```python
from build123d import *

# Parameters (mm, degrees)
SKETCH1_R           = 12.7
BOSS_EXTRUDE1_DEPTH = 1120
SKETCH3_R           = 12.7
SKETCH3_R_2         = 9.525
CUT_EXTRUDE1_DEPTH  = 25.4
SKETCH4_R           = 12.7
SKETCH4_R_2         = 9.525
CUT_EXTRUDE2_DEPTH  = 25.4
SKETCH5_R           = 19.05
SKETCH5_R_2         = 12.7
BOSS_EXTRUDE2_DEPTH = 129


with BuildPart() as part:
    # Sketch1 → Boss-Extrude1 (new body)
    with BuildSketch(Plane(origin=(0, 0, 0), x_dir=(1, 0, 0), z_dir=(0, 1, 0))):
        Circle(SKETCH1_R)
    extrude(amount=BOSS_EXTRUDE1_DEPTH)

    # Sketch3 → Cut-Extrude1 (cut)
    with BuildSketch(Plane.XZ):
        Circle(SKETCH3_R)
        Circle(SKETCH3_R_2, mode=Mode.SUBTRACT)
    extrude(amount=-CUT_EXTRUDE1_DEPTH, mode=Mode.SUBTRACT)

    # Sketch4 → Cut-Extrude2 (cut)
    with BuildSketch(Plane(origin=(0, 1120, 0), x_dir=(1, 0, 0), z_dir=(0, 1, 0))):
        Circle(SKETCH4_R)
        Circle(SKETCH4_R_2, mode=Mode.SUBTRACT)
    extrude(amount=-CUT_EXTRUDE2_DEPTH, mode=Mode.SUBTRACT)

    # Sketch5 → Boss-Extrude2 (add)
    with BuildSketch(Plane(origin=(0, 753, 0), x_dir=(1, 0, 0), z_dir=(0, 1, 0))):
        Circle(SKETCH5_R)
        Circle(SKETCH5_R_2, mode=Mode.SUBTRACT)
    extrude(amount=-BOSS_EXTRUDE2_DEPTH)


solid = part.part
```
Design review of the part built by this model. Coordinates are the model's own, in mm. A direction names the side the tool comes from. Give positions to 0.01 mm unless a question says otherwise; leave off trailing zeros. Loops run counter-clockwise (first coordinate to the right, second up) from the corner with the lowest first, then second, coordinate; pieces in that order, holes last. Notation, with made-up numbers: M -21,80 L 5,80 A28 ccw 5,115 Z; hole C 21,82.25 d3. An arc over 180 degrees is marked long. Return JSON: item names as keys, results as strings. Group by question number.
Item 1: Tool access review of faces 1 (the cylindrical face through (-7.559, 1107.478, 5.796)), 2 (the flat face through (0, 0, 0)), 3 (the flat face through (5, 25.4, 9)): name each direction out of +Z, -Z, +X, -X, +Y, -Y from which nothing blocks a thin tool from reaching the whole face with its end or side.
Item 2: Insertion check: pin 1 Ø12 at (y, z) = (478.5, 7.5) entering from -X; pin 2 Ø1 at (y, z) = (722, -15) entering from +X; pin 3 Ø3 at (x, z) = (13.5, -1.5) entering from +Y. Each pin has a flat end and moves straight along its axis. Give the tip position at first contact, or say it passes through.
Item 3: We need section C-C (y = 1023.5). Give the boundary of the cut face in (x, z).
Item 4: We need section B-B (x = 3). Give the boundary of the cut face in (y, z).
Item 5: For probe 1 along Y at (x, z) = (2, 12.5); probe 2 along Y at (x, z) = (5, -14); probe 3 along X at (y, z) = (613, -1), list the stretches that pass through material, from the lowest coordinate up.
Item 6: We need section A-A (z = 0). Give the boundary of the cut face in (x, y) (3 decimals), and give its area (3 significant figures).
Output:
{
 "1": {"face 1": "+Y", "face 2": "+Z, -Z, +X, -X, -Y", "face 3": "-Y"},
 "2": {"pin 1": "stops at x = -12.61", "pin 2": "stops at x = 12.36", "pin 3": "stops at y = 1094.6"},
 "3": {"outline": "C 0,0 d25.4"},
 "4": {"outline": "M 0,-9.04 L 25.4,-9.04 L 25.4,-12.34 L 624,-12.34 L 624,-18.81 L 753,-18.81 L 753,-12.34 L 1094.6,-12.34 L 1094.6,-9.04 L 1120,-9.04 L 1120,9.04 L 1094.6,9.04 L 1094.6,12.34 L 753,12.34 L 753,18.81 L 624,18.81 L 624,12.34 L 25.4,12.34 L 25.4,9.04 L 0,9.04 Z"},
 "5": {"probe 1": "y = 25.4 to 1094.6", "probe 2": "y = 624 to 753", "probe 3": "x = -12.66 to 12.66"},
 "6": {"outline": "M -19.05,624 L -12.7,624 L -12.7,25.4 L -9.525,25.4 L -9.525,0 L 9.525,0 L 9.525,25.4 L 12.7,25.4 L 12.7,624 L 19.05,624 L 19.05,753 L 12.7,753 L 12.7,1094.6 L 9.525,1094.6 L 9.525,1120 L -9.525,1120 L -9.525,1094.6 L -12.7,1094.6 L -12.7,753 L -19.05,753 Z", "area": "29,800 mm^2"}
}
